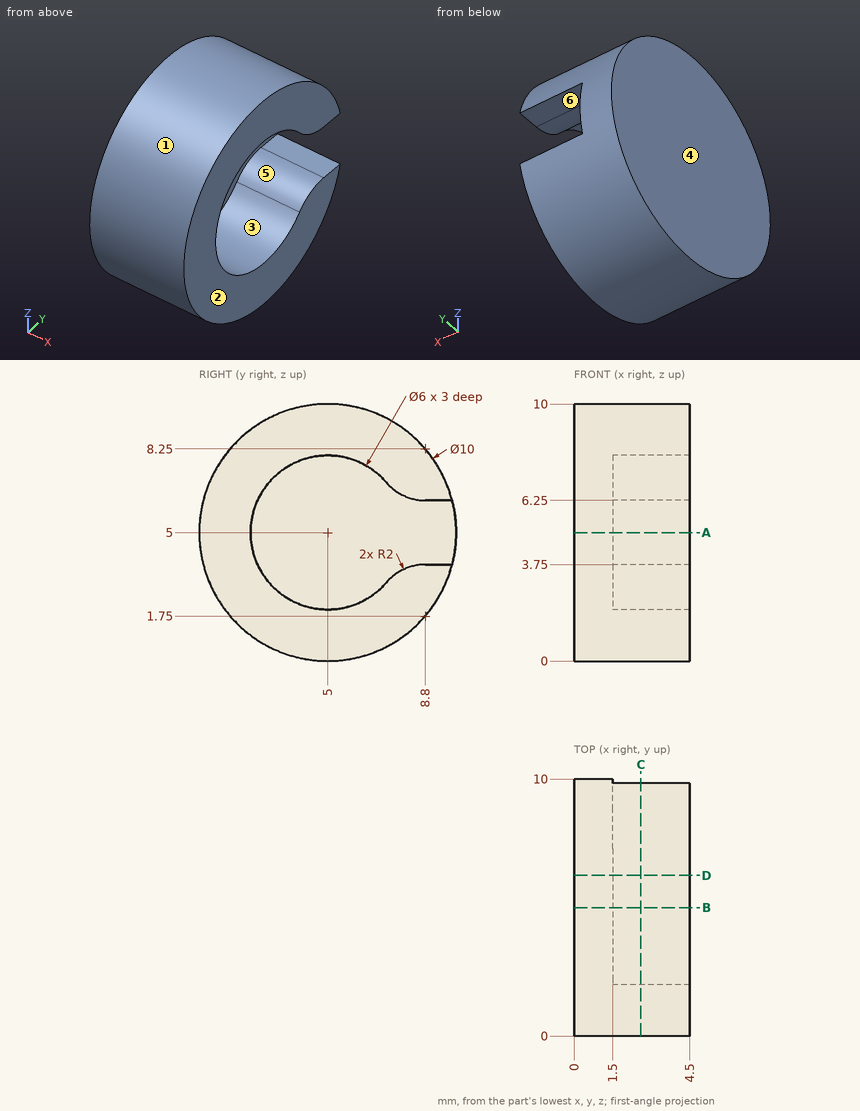
Source: three-view drawing plus pictorial views. Frame: mm from the lowest corner of the part. A direction names the side the tool comes from. Coordinates: 2 decimals unless noted, no trailing zeros. Order: outer loops, then holes, each group sorted by start corner. A loop starts at its lowest first (then second) coordinate and runs counter-clockwise, first axis right, second up. Notation, with made-up numbers: (73, 4) -> (88, 4) arc R20 cw to (88, 29) -> close; hole circle Ø10 at (-11.75, -37). An arc over 180 degrees is marked (long way). Write item = value, one per line.
(1) Cut plane B-B on y = 5. Return loops of the section in (x, z).
Solved:
outline = (0, 0) -> (4.5, 0) -> (4.5, 2) -> (1.5, 2) -> (1.5, 8) -> (4.5, 8) -> (4.5, 10) -> (0, 10) -> close
(2) Pin query (flat end, axial travel): pin 1 Ø2 at (x, y) = (4, 2) entering from -Z; pin 2 Ø5 at (y, z) = (8, 5.5) entering from +X; pin 3 Ø1.5 at (x, y) = (1, 3.5) entering from -Z. Return the tip coordinate at first contact, or that it passes through.
Solved:
pin_1 = 0.42
pin_2 = 4.5
pin_3 = 0.06
(3) Cut plane D-D on y = 6.25. Return loops of the section in (x, z), plus the area to 3 significant figures.
Solved:
outline = (0, 0.16) -> (4.5, 0.16) -> (4.5, 2.27) -> (1.5, 2.27) -> (1.5, 7.73) -> (4.5, 7.73) -> (4.5, 9.84) -> (0, 9.84) -> close
area = 27.2 mm²
(4) Access query for the marked faces 4, 5 and 6. Directions: +Z, -Z, +X, -X, +Y, -Y. A direction counts if a zero-diameter tool reaches every point of the face in a straight line with its end or side. Return the directions, or none.
Solved:
face_4 = +Z, -Z, -X, +Y, -Y
face_5 = +X
face_6 = +X, +Y
(5) Line query: line 1 (Z direction, x = 2.2, y = 5); line 2 (Y direction, x = 2.9, z = 5); line 3 (Z direction, x = 2.25, y = 2.5). Output: solid intervals per line, ascending.
Solved:
line_1 = 0 to 2, 8 to 10
line_2 = 0 to 2
line_3 = 0.67 to 3.34, 6.66 to 9.33
(6) Cut plane A-A on z = 5. Return loops of the section in (x, y).
Solved:
outline = (0, 0) -> (4.5, 0) -> (4.5, 2) -> (1.5, 2) -> (1.5, 10) -> (0, 10) -> close
(7) Cut plane C-C on x = 2.6. Return loops of the section in (y, z).
Solved:
outline = (7.28, 3.05) arc R3 cw (long way) to (7.28, 6.95) arc R2 ccw to (8.8, 6.25) -> (9.84, 6.25) arc R5 ccw (long way) to (9.84, 3.75) -> (8.8, 3.75) arc R2 ccw to start
(8) Pull-direction query (Z, two-part tool) for the marked faces 1, 2 and 3; classes: pulls with the +Z half, pulls with the -Z half, needs draft (parallel to the pull), parting line crosses it, or undercut.
Solved:
face_1 = parting line crosses it
face_2 = needs draft
face_3 = undercut
